```python
from build123d import *

# Parameters (mm, degrees)
F0_W     = 3
F0_H     = 122
F1_DEPTH = 12
F2_W     = 12
F2_H     = 10
F3_DEPTH = 25
F5_DEPTH = 3.001


with BuildPart() as f1:
    # F0 (on Right) → F1 (new body)
    with BuildSketch(Plane.YZ):
        with Locations((-1.5, 61)):
            Rectangle(F0_W, F0_H)
    extrude(amount=F1_DEPTH)

    # F2 (on face) → F3 (join)
    with BuildSketch(Plane(origin=(0, 0, 0), x_dir=(-1, 0, 0), z_dir=(0, 1, 0))):
        with Locations((-6, 5)):
            Rectangle(F2_W, F2_H)
    extrude(amount=F3_DEPTH)

    # F4 (on face) → F5 (cut, through all)
    with BuildSketch(Plane(origin=(0, 0, 0), x_dir=(-1, 0, 0), z_dir=(0, 1, 0))):
        Polygon((-0.5, 118), (-1.5, 118), (-2.5, 118), (-2.5, 48), (-1.5, 48), (-0.5, 48), align=None)
    extrude(amount=-F5_DEPTH, mode=Mode.SUBTRACT)


solid = f1.part
```
Geometry: final body of the model. Coordinates: model frame, mm. A direction names the side the tool comes from. Round coordinates to 2 decimals unless told otherwise and drop trailing zeros. Write each loop counter-clockwise with the first axis right and the second up, starting at its lowest first coordinate (ties: lowest second). Pieces come first, ordered by that corner, then holes. Notation, with made-up numbers: M -16.75,60 L 32.25,60 A19 ccw 32.25,65 Z; hole C 33.5,43.25 d4. An arc over 180 degrees is marked long. Answer in a Markdown table with one row per item. Add a question column.
(1) Cut plane C-C, the plane x = 9. Return the cut outline in (y, z).
(2) Reachability of faces 1 (the face through (6, 12, 10)), 2 (the face through (6, 25, 5)), 3 (the face through (2.5, -1, 83)) from +Z, -Z, +X, -X, +Y, -Y: full face, straight path, thin tool, end or side. Return the list, or none.
(3) Ray query, L1, parallel to Z at x = 3.5, y = 6.75; L2, parallel to Y at x = 5, z = 51. Return the intervals inside material, ascending.
(4) Contact query for flat-ended pins moving along their axis: pin 1 (6 mm diameter, centred on x = 5, z = 64, fed in from +Y); pin 2 (6 mm diameter, centred on x = 6, y = 15.5, fed in from +Z). Output: stop coordinate, or through.
(5) Draft query along Z for faces 4 (the face through (0, -2, 38)), 5 (the face through (6, 11, 0)), 6 (the face through (0.5, -1, 83)). Return one class per face: pulls with the +Z half, pulls with the -Z half, needs draft (parallel to the pull), parting line crosses it, or undercut.
(6) Cut plane D-D, the plane z = 12. Return the cut outline in (x, y), then the cut area to 3 significant figures.
(7) Cut plane B-B, the plane y = 18.75. Return the cut outline in (x, z).
(8) Cut plane A-A, the plane z = 60. Return the cut outline in (x, y).
Established:
| question | item | result |
|---|---|---|
| 1 | outline | M -3,0 L 25,0 L 25,10 L 0,10 L 0,122 L -3,122 Z |
| 2 | face 1 | +Z, +X, -X, +Y |
| 2 | face 2 | +Z, -Z, +X, -X, +Y |
| 2 | face 3 | +Y, -Y |
| 3 | L1 | 0 to 10 |
| 3 | L2 | -3 to 0 |
| 4 | pin 1 | y = 0 |
| 4 | pin 2 | z = 10 |
| 5 | face 4 | needs draft |
| 5 | face 5 | pulls with the -Z half |
| 5 | face 6 | undercut |
| 6 | outline | M 0,-3 L 12,-3 L 12,0 L 0,0 Z |
| 6 | area | 36.0 mm² |
| 7 | outline | M 0,0 L 12,0 L 12,10 L 0,10 Z |
| 8 | outline | M 0,-3 L 0.5,-3 L 0.5,0 L 0,0 Z; M 2.5,-3 L 12,-3 L 12,0 L 2.5,0 Z |
